Input: dimensioned drawing with shaded views. Units: mm. Origin: part minimum x, y, z. A direction names the side the tool comes from. Coordinates: 2 decimals unless noted, no trailing zeros. Loops run counter-clockwise (first coordinate to the right, second up) from the corner with the lowest first, then second, coordinate; pieces in that order, holes last. Notation, with made-up numbers: (-35, 6.5) - (-29, 6.5) arc R29 cw to (-29, 28.5) - close; hole circle Ø10 at (-11, 3.5). An arc over 180 degrees is marked (long way). Write item = value, one per line. Start each with the question number.
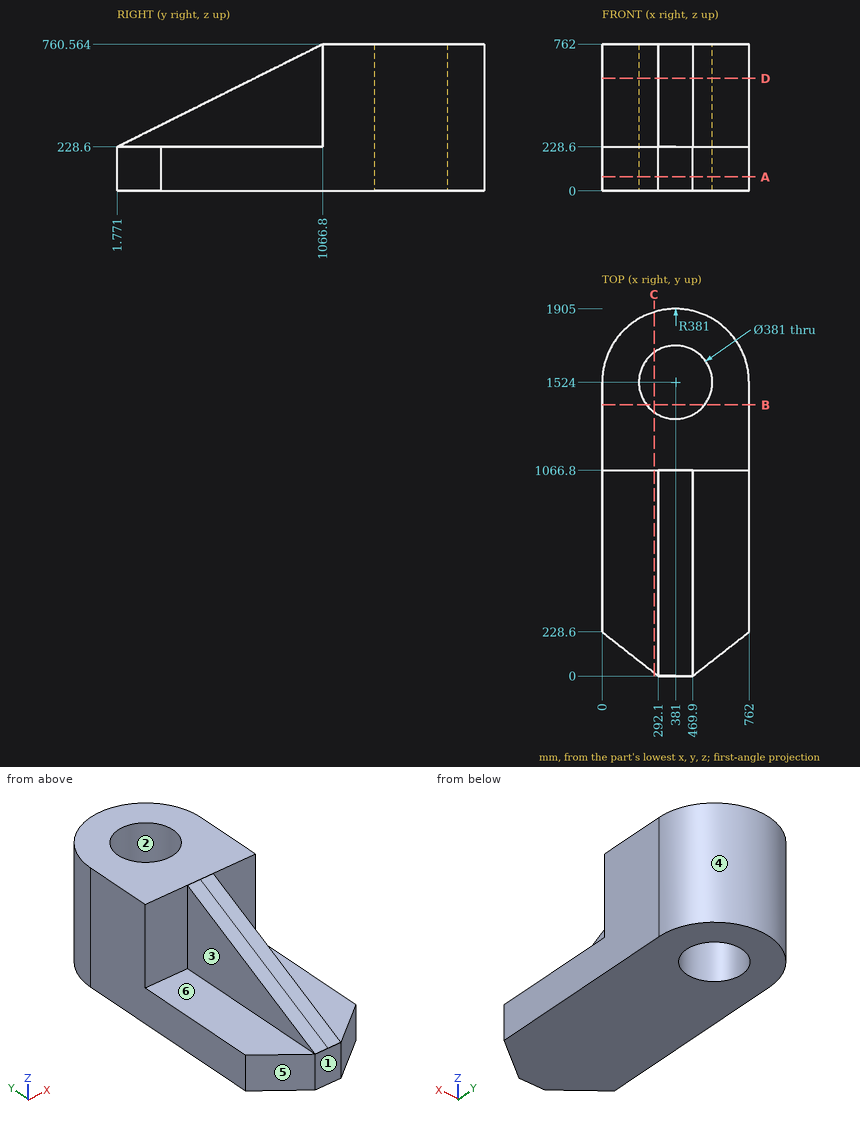
Item 1: Cut plane D-D on z = 583. Return loops of the section in (x, y).
Item 2: Cut plane B-B on y = 1407. Return loops of the section in (x, z), plus the area to 3 significant figures.
Item 3: Cut plane A-A on z = 72.5. Return loops of the section in (x, y).
Item 4: Pin query (flat end, axial travel): pin 1 (12 mm diameter, centred on x = 465, y = 724.5, fed in from +Z); pin 2 (1.5 mm diameter, centred on x = 475.5, z = 508, fed in from -Y); pin 3 (8 mm diameter, centred on x = 280.5, z = 160, fed in from +Y). Return the tip coordinate at first contact, or that it passes through.
Item 5: Pull-direction query (X, two-part tool) for the marked faces 1, 2, 3 and 4; classes: pulls with the +X half, pulls with the -X half, needs draft (parallel to the pull), parting line crosses it, or undercut.
Item 6: Access query for the marked faces 5 and 6. Directions: +Z, -Z, +X, -X, +Y, -Y. A direction counts if a zero-diameter tool reaches every point of the face in a straight line with its end or side. Return the directions, or none.
Item 7: Cut plane C-C on x = 270. Return loops of the section in (y, z), plus the area to 3 significant figures.
Item 8: Ray query, line 1 (Y direction, x = 392.5, z = 36); line 2 (Z direction, x = 561, y = 125); line 3 (X direction, y = 634, z = 424). Return the intervals inside material, ascending.
Recorded:
q1.outline = (0, 1066.8) - (292.1, 1066.8) - (292.1, 711.3) - (469.9, 711.3) - (469.9, 1066.8) - (762, 1066.8) - (762, 1524) arc R381 ccw to (0, 1524) - close; hole circle Ø381 at (381, 1524)
q2.outline = (0, 0) - (230.66, 0) - (230.66, 762) - (0, 762) - close; (531.34, 0) - (762, 0) - (762, 762) - (531.34, 762) - close
q2.area = 352,000 mm²
q3.outline = (0, 228.6) - (292.1, 0) - (469.9, 0) - (762, 228.6) - (762, 1524) arc R381 ccw to (0, 1524) - close; hole circle Ø381 at (381, 1524)
q4.pin_1 = 592.59
q4.pin_2 = 1066.8
q4.pin_3 = 1892.58
q5.face_1 = needs draft
q5.face_2 = undercut
q5.face_3 = pulls with the -X half
q5.face_4 = parting line crosses it
q6.face_5 = +Z, -Z, -X, -Y
q6.face_6 = +Z, -Y
q7.outline = (17.3, 0) - (1369.18, 0) - (1369.18, 762) - (1066.8, 762) - (1066.8, 228.6) - (17.3, 228.6) - close; (1678.82, 0) - (1888.47, 0) - (1888.47, 762) - (1678.82, 762) - close
q7.area = 630,000 mm²
q8.line_1 = 0 to 1333.85, 1714.15 to 1904.83
q8.line_2 = 0 to 228.6
q8.line_3 = 292.1 to 469.9
